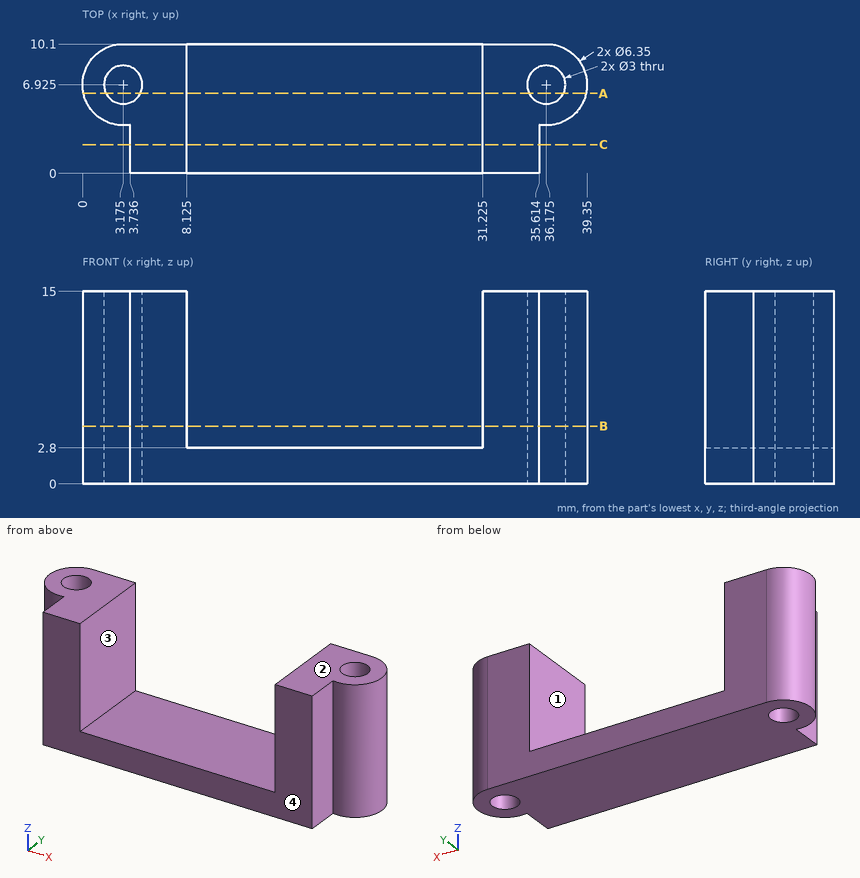
Job drawing, mm, ordinate dimensions from the low corner. One solid piece. A direction names the side the tool comes from. Round coordinates to 2 decimals unless told otherwise and drop trailing zeros. Write each loop counter-clockwise with the first axis right and the second up, starting at its lowest first coordinate (ties: lowest second). Pieces come first, ordered by that corner, then holes. Notation, with made-up numbers: (12, 2) -> (57, 2) arc R20 cw to (57, 35) -> close; hole circle Ø7 at (-33, 0). An arc over 180 degrees is marked (long way). Answer as a JSON object with one key per item and string values.
(1) Band-saw the part on A-A, the plane y = 6.25. List the corners of the cut face in (x, z) (1 decimal), then the cut area to 3 significant figures.
Reported:
{"outline": "(0.1, 0) -> (1.8, 0) -> (1.8, 15) -> (0.1, 15) -> close; (4.5, 0) -> (34.8, 0) -> (34.8, 15) -> (31.2, 15) -> (31.2, 2.8) -> (8.1, 2.8) -> (8.1, 15) -> (4.5, 15) -> close; (37.5, 0) -> (39.3, 0) -> (39.3, 15) -> (37.5, 15) -> close", "area": "226 mm^2"}
(2) Band-saw the part on C-C, the plane y = 2.25. List the corners of the cut face in (x, z) (1 decimal).
Reported:
{"outline": "(3.7, 0) -> (35.6, 0) -> (35.6, 15) -> (31.2, 15) -> (31.2, 2.8) -> (8.1, 2.8) -> (8.1, 15) -> (3.7, 15) -> close"}
(3) Pin check, flat tips, straight feed: P1, Ø1.1, axis at y = 1, z = 5.5, coming from the -X side; P2, Ø3, axis at y = 2.5, z = 11, coming from the +X side; P3, Ø1.5, axis at y = 5.5, z = 5, coming from the -X side. Stop position of each tip, or through.
Reported:
{"P1": "stops at x = 3.74", "P2": "stops at x = 37.41", "P3": "stops at x = 0.07"}
(4) Two-plate mould, pull along X, no slides. Class the marked faces 1 and 2: +X half, -X half, draft (parallel to the pull), parting line (faces both ways), or undercut.
Reported:
{"face 1": "undercut", "face 2": "draft"}
(5) Probe probe 1 along X at (y, z) = (7, 1.75); probe 2 along X at (y, z) = (7, 6) (1 decimal); probe 3 along X at (y, z) = (6.5, 3) (1 decimal). List the from-to ranges inside material, lowest first. Write a range as [from, to].
Reported:
{"probe 1": "x = [0, 1.68], [4.67, 34.68], [37.67, 39.35]", "probe 2": "x = [0, 1.7], [4.7, 8.1], [31.2, 34.7], [37.7, 39.3]", "probe 3": "x = [0, 1.7], [4.6, 8.1], [31.2, 34.7], [37.6, 39.3]"}
(6) Which spindle directions (+Z, -Z, +X, -X, +Y, -Y) get a long thin tool onto all of the face, cutting with end or side? Do the marked faces 3 and 4. Say none if no direction does.
Reported:
{"face 3": "+Z, +Y, -Y", "face 4": "+Z, -Z, +X, -X, -Y"}
(7) Band-saw the part on B-B, the plane z = 4.5. Count the separate pieces of the cut face and the enclosed holes in it, then the cut area to 3 significant figures.
Reported:
{"separate pieces": "2", "enclosed holes": "2", "area": "113 mm^2"}
